Verification items for the finished model (mm, model axes). A direction names the side the tool comes from. Give positions to 0.01 mm unless a question says otherwise; leave off trailing zeros. Order: outer loops, then holes, each group sorted by start corner. A loop starts at its lowest first (then second) coordinate and runs counter-clockwise, first axis right, second up. Notation, with made-up numbers: (54.25, 53) -> (100.25, 53) arc R21 ccw to (100.25, 92) -> close; hole circle Ø1 at (-33.75, -16). An arc over 180 degrees is marked (long way). Return JSON: item names as keys, results as strings. Group by question number.
(1) Cross-section at D-D on x = 58. Enter the section's corners in (y, z), then the cut area to 3 significant figures.
(2) Depth check by flat-ended pin: pin 1 Ø4 at (x, y) = (29.4, -40) entering from -Z; pin 2 Ø2.5 at (y, z) = (-36, -1) entering from +X; pin 3 Ø1 at (x, y) = (1.5, -20) entering from +Z. Enter the tip coordinate at first touch or a pass-through.
(3) Tool access check on faces 5 (the face through (98, -30, -3)), 6 (the face through (85.6, -30, -1)), 7 (the face through (2, -30, -3)), 8 (the face through (7, -30, 0)). Record the directions out of +Z, -Z, +X, -X, +Y, -Y that give a thin tool (end or side, any length) a straight path to the whole face; none if there is none.
(4) Cross-section at A-A on z = -1.5. State how many separate pieces and enclosed holes the cut face has, then the cut area to 3 significant figures.
(5) Cross-section at B-B on x = 74.4. Enter the section's corners in (y, z).
(6) Thickness scan on line 1 along Y through (x, z) = (74.4, -1.05); line 2 along X through (y, z) = (-29.5, -3.5); line 3 along X through (y, z) = (-36.5, -2.1). Record the ranges inside material, lowest first.
(7) Release check for a two-part mould opening along Y. For faces 1 (the face through (49, 0, -2)), 2 (the face through (30.74, -17.89, -2.46)), 3 (the face through (68.406, -29.736, -2.465)), 4 (the face through (87, -30, -3)) record: pulls with the +Y half, pulls with the -Y half, needs draft (parallel to the pull), parting line crosses it, or undercut.
from build123d import *

# Parameters (mm, degrees)
F0_W     = 100
F0_H     = 60
F1_DEPTH = 5
F2_W     = 3.2
F2_H     = 60
F3_DEPTH = 3
F4_R     = 6
F4_R_2   = 2.5
F5_DEPTH = 5


with BuildPart() as f1:
    # F0 (on Top) → F1 (new body)
    with BuildSketch(Plane.XY):
        with Locations((50, -30)):
            Rectangle(F0_W, F0_H)
    extrude(amount=-F1_DEPTH)

    # F2 (on face) → F3 (cut)
    with BuildSketch(Plane.XY):
        with Locations((1.6, -30)):
            Rectangle(F2_W, F2_H)
        with Locations((12.8, -30)):
            Rectangle(F2_W, F2_H)
        with Locations((87.2, -30)):
            Rectangle(F2_W, F2_H)
        with Locations((98.4, -30)):
            Rectangle(F2_W, F2_H)
    extrude(amount=-F3_DEPTH, mode=Mode.SUBTRACT)

    # F4 (on face) → F5 (cut)
    with BuildSketch(Plane.XY):
        with Locations((29.4, -50)):
            Circle(F4_R)
        with Locations((44.4, -50)):
            Circle(F4_R)
        with Locations((59.4, -50)):
            Circle(F4_R)
        with Locations((74.4, -50)):
            Circle(F4_R)
        with Locations((74.4, -40)):
            Circle(F4_R_2)
        with Locations((59.4, -40)):
            Circle(F4_R_2)
        with Locations((44.4, -40)):
            Circle(F4_R_2)
        with Locations((29.4, -40)):
            Circle(F4_R_2)
        with Locations((29.4, -30)):
            Circle(F4_R)
        with Locations((44.4, -30)):
            Circle(F4_R)
        with Locations((59.4, -30)):
            Circle(F4_R)
        with Locations((74.4, -30)):
            Circle(F4_R)
        with Locations((74.4, -20)):
            Circle(F4_R_2)
        with Locations((59.4, -20)):
            Circle(F4_R_2)
        with Locations((44.4, -20)):
            Circle(F4_R_2)
        with Locations((29.4, -20)):
            Circle(F4_R_2)
        with Locations((74.4, -10)):
            Circle(F4_R)
        with Locations((59.4, -10)):
            Circle(F4_R)
        with Locations((44.4, -10)):
            Circle(F4_R)
        with Locations((29.4, -10)):
            Circle(F4_R)
    extrude(amount=-F5_DEPTH, mode=Mode.SUBTRACT)


solid = f1.part
Verdict:
{
 "1": {"outline": "(-60, -5) -> (-55.83, -5) -> (-55.83, 0) -> (-60, 0) -> close; (-44.17, -5) -> (-42.07, -5) -> (-42.07, 0) -> (-44.17, 0) -> close; (-37.93, -5) -> (-35.83, -5) -> (-35.83, 0) -> (-37.93, 0) -> close; (-24.17, -5) -> (-22.07, -5) -> (-22.07, 0) -> (-24.17, 0) -> close; (-17.93, -5) -> (-15.83, -5) -> (-15.83, 0) -> (-17.93, 0) -> close; (-4.17, -5) -> (0, -5) -> (0, 0) -> (-4.17, 0) -> close", "area": "83.5 mm²"},
 "2": {"pin 1": "through", "pin 2": "x = 96.8", "pin 3": "z = -3"},
 "3": {"face 5": "+Z, +X, +Y, -Y", "face 6": "+Z, +Y, -Y", "face 7": "+Z, -X, +Y, -Y", "face 8": "+Z, +X, -X, +Y, -Y"},
 "4": {"separate pieces": "3", "enclosed holes": "20", "area": "3,720 mm²"},
 "5": {"outline": "(-60, -5) -> (-56, -5) -> (-56, 0) -> (-60, 0) -> close; (-44, -5) -> (-42.5, -5) -> (-42.5, 0) -> (-44, 0) -> close; (-37.5, -5) -> (-36, -5) -> (-36, 0) -> (-37.5, 0) -> close; (-24, -5) -> (-22.5, -5) -> (-22.5, 0) -> (-24, 0) -> close; (-17.5, -5) -> (-16, -5) -> (-16, 0) -> (-17.5, 0) -> close; (-4, -5) -> (0, -5) -> (0, 0) -> (-4, 0) -> close"},
 "6": {"line 1": "-60 to -56, -44 to -42.5, -37.5 to -36, -24 to -22.5, -17.5 to -16, -4 to 0", "line 2": "0 to 23.42, 35.38 to 38.42, 50.38 to 53.42, 65.38 to 68.42, 80.38 to 100", "line 3": "3.2 to 11.2, 14.4 to 85.6, 88.8 to 96.8"},
 "7": {"face 1": "pulls with the +Y half", "face 2": "undercut", "face 3": "undercut", "face 4": "needs draft"}
}
